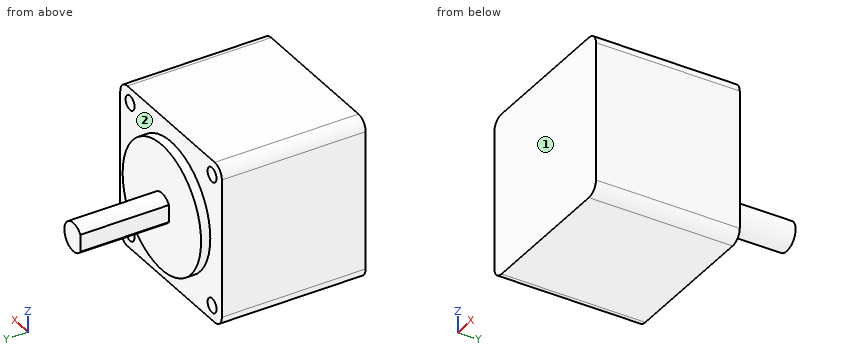
Autodesk Inventor part; units mm, degrees
ref_plane "YZ Plane" through (0, 0, 0) normal (1, 0, 0) x (0, 1, 0)
ref_plane "XZ Plane" through (0, 0, 0) normal (0, 1, 0) x (-1, 0, 0)
ref_plane "XY Plane" through (0, 0, 0) normal (0, 0, 1) x (1, 0, 0)
sketch "草圖1" plane through (0, 0, 0) normal (0, 1, 0) x (-1, 0, 0)
  line L0 (-14.25, 14.075) -> (14.25, 14.075)
  line L1 (14.25, 14.075) -> (14.25, -14.075)
  line L2 (14.25, -14.075) -> (-14.25, -14.075)
  line L3 (-14.25, -14.075) -> (-14.25, 14.075)
  line L4 (-14.25, 14.075) -> (14.25, -14.075) construction
  line L5 (14.25, 14.075) -> (-14.25, -14.075) construction
  point P0 (0, 0)
  dimension "d0" = 28.5
  dimension "d1" = 28.15
extrude "擠出1" add sketch "草圖1" along normal blind 25
sketch "草圖2" plane through (0, 25, 0) normal (0, 1, 0) x (1, 0, 0)
  circle A0 centre (0, 0) radius 11
  dimension "d4" = 22
extrude "擠出2" add sketch "草圖2" along normal blind 1.6
sketch "草圖3" plane through (0, 26.6, 0) normal (0, 1, 0) x (1, 0, 0)
  arc A0 (-2, -1.5) -> (-2, 1.5) centre (0, 0) ccw
  line L0 (-2, -1.5) -> (-2, 1.5)
  dimension "d7" = 5
  dimension "d8" = 2
extrude "擠出3" add sketch "草圖3" along normal blind 15.4
sketch "草圖4" plane through (0, 25, 0) normal (0, 1, 0) x (1, 0, 0)
  line L0 (11.5, -11.5) -> (-11.5, -11.5) construction
  line L1 (-11.5, -11.5) -> (-11.5, 11.5) construction
  line L2 (-11.5, 11.5) -> (11.5, 11.5) construction
  line L3 (11.5, 11.5) -> (11.5, -11.5) construction
  arc A0 (-2, -1.5) -> (-2, 1.5) centre (0, 0) ccw construction
  line L4 (11.5, -11.5) -> (-11.5, 11.5) construction
  line L5 (-11.5, -11.5) -> (11.5, 11.5) construction
  circle A1 centre (-11.5, 11.5) radius 1.25
  circle A2 centre (-11.5, -11.5) radius 1.25
  circle A3 centre (11.5, -11.5) radius 1.25
  circle A4 centre (11.5, 11.5) radius 1.25
  dimension "d11" = 23
  dimension "d12" = 23
  dimension "d13" = 2.5
  dimension "d16" = 360
extrude "擠出4" cut sketch "草圖4" against normal blind 3.5
fillet "圓角1" radius 2 4 edges at (14.25, 12.5, 14.075) (14.25, 12.5, -14.075) (-14.25, 12.5, 14.075) (-14.25, 12.5, -14.075)
sketch "草圖5" plane through (0, 42, 0) normal (0, 1, 0) x (1, 0, 0)
  point P0 (0, 0)
  point P1 (0, 0)
properties part number "nema 11x25"
Geometry: final body of the model. Coordinates: model frame, mm. Face numbers are marked on the shaded views. A direction names the side the tool comes from. Round coordinates to 2 decimals unless told otherwise and drop trailing zeros. Write each loop counter-clockwise with the first axis right and the second up, starting at its lowest first coordinate (ties: lowest second). Pieces come first, ordered by that corner, then holes. Notation, with made-up numbers: (-15.75, -27) -> (30.25, -27) arc R14 ccw to (30.25, -20) -> close; hole circle Ø9 at (20.25, 49.5). An arc over 180 degrees is marked (long way). Return JSON: item names as keys, results as strings.
Q1. Section C-C on y = 27.5. Return the cut outline in (x, z), and give its area (3 significant figures).
From the geometry:
{"outline": "(-2, -1.5) arc R2.5 ccw (long way) to (-2, 1.5) -> close", "area": "18.6 mm2"}
Q2. Ray query, line 1 (Z direction, x = -11.5, y = 23.55) (3 decimals); line 2 (X direction, y = 22.85, z = -11.5); line 3 (Y direction, x = 12, z = 3.75). Return the intervals inside material, ascending.
From the geometry:
{"line 1": "-14.075 to -12.75, -10.25 to 10.25, 12.75 to 14.075", "line 2": "-14.25 to -12.75, -10.25 to 10.25, 12.75 to 14.25", "line 3": "0 to 25"}
Q3. Section D-D on x = -4. Return the cut outline in (y, z) (3 decimals), and give its area (3 significant figures).
From the geometry:
{"outline": "(0, -14.075) -> (25, -14.075) -> (25, -10.247) -> (26.6, -10.247) -> (26.6, 10.247) -> (25, 10.247) -> (25, 14.075) -> (0, 14.075) -> close", "area": "737 mm2"}
Q4. Section B-B on z = -11.5. Return the cut outline in (x, y), and give its area (3 significant figures).
From the geometry:
{"outline": "(-14.25, 0) -> (14.25, 0) -> (14.25, 25) -> (12.75, 25) -> (12.75, 21.5) -> (10.25, 21.5) -> (10.25, 25) -> (-10.25, 25) -> (-10.25, 21.5) -> (-12.75, 21.5) -> (-12.75, 25) -> (-14.25, 25) -> close", "area": "695 mm2"}
Q5. Set-up query: the marked faces 1 and 2. Return all of +Z, -Z, +X, -X, +Y, -Y with unobstructed straight access to the full face (end or side cutting, diameter ignored); none if empty.
From the geometry:
{"face 1": "+Z, -Z, +X, -X, -Y", "face 2": "+Y"}
Q6. First-contact query: pin 1 Ø2 at (x, z) = (-11.5, -11.5) entering from +Y; pin 2 Ø8.5 at (x, z) = (-0.5, 2.5) entering from +Y; pin 3 Ø3 at (x, z) = (-11.5, 11.5) entering from +Y; pin 4 Ø1.5 at (y, z) = (36.5, 0.5) entering from -X. Flat tips, straight axial feed; report the tip coordinate or a pass-through.
From the geometry:
{"pin 1": "y = 21.5", "pin 2": "y = 42", "pin 3": "y = 25", "pin 4": "x = -2"}
Q7. Section A-A on x = 11.5. Return the cut outline in (y, z) (3 decimals).
From the geometry:
{"outline": "(0, -14.075) -> (25, -14.075) -> (25, -12.75) -> (21.5, -12.75) -> (21.5, -10.25) -> (25, -10.25) -> (25, 10.25) -> (21.5, 10.25) -> (21.5, 12.75) -> (25, 12.75) -> (25, 14.075) -> (0, 14.075) -> close"}
